Here's how the part is built. I have some questions about the finished solid (model axes, mm). A direction names the side the tool comes from. Coordinates: 2 decimals unless noted, no trailing zeros. Order: outer loops, then holes, each group sorted by start corner. A loop starts at its lowest first (then second) coordinate and runs counter-clockwise, first axis right, second up. Notation, with made-up numbers: (56.25, 20) - (68.25, 20) arc R24 ccw to (68.25, 55) - close; hole circle Ø7 at (-12, 30.25). An arc over 180 degrees is marked (long way). Use one line per item in the form item = value. Start each with the question number.
from build123d import *

# Parameters (mm, degrees)
F0_W     = 304.8
F0_H     = 762
F0_W_2   = 19.05
F0_H_2   = 406.4
F1_DEPTH = 6.35


with BuildPart() as f1:
    # F0 (on Right) → F1 (new body, symmetric)
    with BuildSketch(Plane.YZ):
        with Locations((152.4, 381)):
            Rectangle(F0_W, F0_H)
        with Locations((152.4, 330.2)):
            Rectangle(F0_W_2, F0_H_2, mode=Mode.SUBTRACT)
    extrude(amount=F1_DEPTH, both=True)


solid = f1.part
1) If we mould it in two halves opening along Z, with no side actions, what happens to faces 3 (the flat face through (6.35, 184, 386)), 4 (the flat face through (0, 150, 762)), 5 (the flat face through (0, 142.875, 327))? For each: pulls with the +Z half, pulls with the -Z half, needs draft (parallel to the pull), parting line crosses it, or undercut.
2) I need wall thicknesses on probe 1 along Y at (x, z) = (-5.5, 429) (3 decimals); probe 2 along Z at (x, y) = (-4.5, 144). Which ranges of each line are inside material? Lowest first, please. Write a range as [from, to].
3) Suppose I cut it at B-B, the plane x = 2. List the corners of the cut face in (y, z) for me (3 decimals).
4) Suppose I cut it at A-A, the plane z = 321.5. List the corners of the cut face in (x, y) for me (3 decimals), then the cut area to 3 significant figures.
5) Which directions (+Z, -Z, +X, -X, +Y, -Y) give clear straight access to the entire face, cutting with the end or side of a thin tool? Please do faces 1 (the flat face through (0, 152, 127)), 2 (the flat face through (-6.35, 184, 386)).
From the geometry:
q1.face_3 = needs draft
q1.face_4 = pulls with the +Z half
q1.face_5 = undercut
q2.probe_1 = [0, 142.875], [161.925, 304.8]
q2.probe_2 = [0, 127], [533.4, 762]
q3.outline = (0, 0) - (304.8, 0) - (304.8, 762) - (0, 762) - close; hole (142.875, 127) - (161.925, 127) - (161.925, 533.4) - (142.875, 533.4) - close
q4.outline = (-6.35, 0) - (6.35, 0) - (6.35, 142.875) - (-6.35, 142.875) - close; (-6.35, 161.925) - (6.35, 161.925) - (6.35, 304.8) - (-6.35, 304.8) - close
q4.area = 3,630 mm2
q5.face_1 = +X, -X
q5.face_2 = +Z, -Z, -X, +Y, -Y
